```python
from build123d import *

# Parameters (mm, degrees)
F1_DEPTH  = 275.93
F3_DEPTH  = 255.93
F9_OFFSET = 0.125


with BuildPart() as f1:
    # F0 (on Front) → F1 (new body)
    with BuildSketch(Plane.XZ):
        with BuildLine():
            Line((-14.5, 0), (-14.5, -25.5))
            ThreePointArc((-14.5, -25.5), (-10.2530483272, -35.7530483272), (0, -40))
            ThreePointArc((0, -40), (10.2530483272, -35.7530483272), (14.5, -25.5))
            Line((14.5, -25.5), (14.5, 0))
            Line((14.5, 0), (-14.5, 0))
        make_face()
    extrude(amount=-F1_DEPTH)


with BuildPart() as f3:
    # F2 (on Front) → F3 (new body)
    with BuildSketch(Plane.XZ):
        Polygon((0, -4.5), (0, 3.5), (-3, 3.5), (-3, 2), (-8, 2), (-8, -3), (-3, -3), (-3, -4.5), align=None)
    extrude(amount=-F3_DEPTH)


with BuildPart() as f3_1:
    # F4: moved
    add(f3.part.moved(Location((-8.5, 5, -9))))


with BuildPart() as f6:
    # F5 (on Front) → F6 (revolve)
    with BuildSketch(Plane.XZ):
        Polygon((3, 5), (0, 5), (0, 0), (3, 0), (8, 0), (8, 3), (3, 3), align=None)
    revolve(axis=Axis((1.5, 0, 0), (1, 0, 0)))


with BuildPart() as f6_1:
    # F7: moved
    add(f6.part.moved(Location((8.5, 259.93, -9.5))))


with BuildPart() as f8_1:
    # F8: instance of F3
    add(f3_1.part.mirror(Plane.YZ))


with BuildPart() as f8_2:
    # F8: instance of F6
    add(f6_1.part.mirror(Plane.YZ))


with BuildPart() as f1_1:
    add(f1.part)

    # F9: cut F8_1, F3, F6, F8_2, each made larger all round first
    f9_tool = offset(f8_1.part, amount=F9_OFFSET, kind=Kind.INTERSECTION, mode=Mode.PRIVATE)
    add(f9_tool, mode=Mode.SUBTRACT)
    f9_tool1 = offset(f3_1.part, amount=F9_OFFSET, kind=Kind.INTERSECTION, mode=Mode.PRIVATE)
    add(f9_tool1, mode=Mode.SUBTRACT)
    f9_tool2 = offset(f6_1.part, amount=F9_OFFSET, kind=Kind.INTERSECTION, mode=Mode.PRIVATE)
    add(f9_tool2, mode=Mode.SUBTRACT)
    f9_tool3 = offset(f8_2.part, amount=F9_OFFSET, kind=Kind.INTERSECTION, mode=Mode.PRIVATE)
    add(f9_tool3, mode=Mode.SUBTRACT)


solid = f1_1.part
```
Check sheet for the modelled part. Datum: model origin and axes. Units: mm. A direction names the side the tool comes from. Round coordinates to 2 decimals unless told otherwise and drop trailing zeros. Order: outer loops, then holes, each group sorted by start corner. A loop starts at its lowest first (then second) coordinate and runs counter-clockwise, first axis right, second up. Notation, with made-up numbers: M -33.5,-24 L -9.5,-24 A32 cw -9.5,15 Z; hole C 34,81.25 d10. An arc over 180 degrees is marked long. Answer in a Markdown table with one row per item.
(1) Gauge pin test, flat ends, axial feed: pin 1 (11.5 mm diameter, centred on y = 147.5, z = -11, fed in from +X); pin 2 (3 mm diameter, centred on x = 4.5, y = 162.5, fed in from -Z); pin 3 (5.5 mm diameter, centred on y = 259.93, z = -9.5, fed in from -X) (3 decimals); pin 4 (3.5 mm diameter, centred on x = 10.5, y = 171.5, fed in from -Z). Record the tip position at first contact, or that the pin passes through.
Findings:
| item | result |
|---|---|
| pin 1 | stops at x = 14.5 |
| pin 2 | stops at z = -39.69 |
| pin 3 | stops at x = -8.375 |
| pin 4 | stops at z = -37.06 |
(2) Draft check along Y on faces 1 (the flat face through (11.625, 134, -6)), 2 (the flat face through (0, 275.93, -20)), 3 (the cylindrical face through (-13.042, 263.054, -9.594)), 4 (the flat face through (14.5, 136, -13)). Enter one of: +Y half, -Y half, draft (parallel to the pull), parting line (faces both ways), or undercut.
Findings:
| item | result |
|---|---|
| face 1 | undercut |
| face 2 | +Y half |
| face 3 | undercut |
| face 4 | draft |
(3) Section check C-C on z = -36. Record the boundary of the cut face in (x, y).
Findings:
| item | result |
|---|---|
| outline | M -10,0 L 10,0 L 10,275.93 L -10,275.93 Z |
(4) Section check A-A on y = 103.5. Record the boundary of the cut face in (x, z) (3 decimals).
Findings:
| item | result |
|---|---|
| outline | M -14.5,-25.5 A14.5 ccw 14.5,-25.5 L 14.5,-12.125 L 11.625,-12.125 L 11.625,-13.625 L 8.375,-13.625 L 8.375,-5.375 L 11.625,-5.375 L 11.625,-6.875 L 14.5,-6.875 L 14.5,0 L -14.5,0 L -14.5,-6.875 L -11.625,-6.875 L -11.625,-5.375 L -8.375,-5.375 L -8.375,-13.625 L -11.625,-13.625 L -11.625,-12.125 L -14.5,-12.125 Z |
(5) Material ranges on line 1 along X through (y, z) = (61, -13) (3 decimals); line 2 along Y through (x, z) = (9.2, -9.5) (3 decimals); line 3 along Y through (x, z) = (12.95, -9.5) (3 decimals), recorded low to high. Write a range as from..to.
Findings:
| item | result |
|---|---|
| line 1 | x = -14.5..-11.625, -8.375..8.375, 11.625..14.5 |
| line 2 | y = 0..4.875, 265.055..275.93 |
| line 3 | y = 0..4.875, 263.055..275.93 |
(6) Set-up check for faces 5 (the flat face through (-11, 4.875, -9)), 6 (the flat face through (0, 0, -20)), 7 (the cylindrical face through (13.042, 263.054, -9.594)): record each of +Z, -Z, +X, -X, +Y, -Y from which the full face is reachable in a straight line by a thin tool's end or side.
Findings:
| item | result |
|---|---|
| face 5 | none |
| face 6 | +Z, -Z, +X, -X, -Y |
| face 7 | +X |
(7) Section check B-B on z = -9.5. Record the boundary of the cut face in (x, y) (3 decimals), plus the area to 3 significant figures.
Findings:
| item | result |
|---|---|
| outline | M -14.5,0 L 14.5,0 L 14.5,4.875 L 8.375,4.875 L 8.375,265.055 L 11.625,265.055 L 11.625,263.055 L 14.5,263.055 L 14.5,275.93 L -14.5,275.93 L -14.5,263.055 L -11.625,263.055 L -11.625,265.055 L -8.375,265.055 L -8.375,4.875 L -14.5,4.875 Z |
| area | 4,830 mm^2 |
